CAD build for the part. Positions are in the model's coordinates, mm. A direction names the side the tool comes from. Round coordinates to 2 decimals unless told otherwise and drop trailing zeros. Order: outer loops, then holes, each group sorted by start corner. A loop starts at its lowest first (then second) coordinate and runs counter-clockwise, first axis right, second up. Notation, with made-up numbers: (59.25, 72) -> (100.25, 72) arc R27 ccw to (100.25, 106) -> close; hole circle Ø4 at (34.25, 85). An arc over 180 degrees is marked (long way). Return JSON: item names as keys, results as strings. Group by question number.
Q1. Probe line 1 along X through (y, z) = (62.5, -68.15); line 2 along Y through (x, z) = (35, -67.9); line 3 along Y through (x, z) = (41, -63.1). List the from-to ranges inside material, lowest first.
Q2. Mould opens along Y. For faces 6 (the flat face through (40, 1, -67)), 7 (the cylindrical face through (-35.962, 64.447, -66.014)), 8 (the cylindrical face through (-93, 62.6, -68.5)) say: +Y half, -Y half, draft (parallel to the pull), parting line (faces both ways), or undercut.
Q3. Cut at D-D (x = -27.5). Write the cut outline in (y, z), then the cut area to 3 significant figures.
Q4. Cut at C-C (x = 41). Write the cut outline in (y, z).
Q5. Cut at B-B (y = 68.5). Write the cut outline in (x, z), then the cut area to 3 significant figures.
Q6. Flat gauge pins, fed straight in: pin 1 (5.5 mm diameter, centred on x = 41, y = -68.5, fed in from +Z); pin 2 (5 mm diameter, centred on x = -90, y = 62.5, fed in from -Z); pin 3 (2 mm diameter, centred on x = 16, y = -37.5, fed in from +Z). Where does each tip first touch, or does it go through?
Q7. Which spindle directions (+Z, -Z, +X, -X, +Y, -Y) get a long thin tool onto all of the face, cutting with end or side? Do faces 1 (the flat face through (40, 1, -65)), 2 (the cylindrical face through (38.6, -70.3, -63.5)), 3 (the cylindrical face through (-71.722, 40.551, -66.028)), 4 (the flat face through (-63, 53, -62)), 5 (the cylindrical face through (-93, -62.4, -68.5)). Say none if no direction does.
Q8. Cut at A-A (y = 0). Write the cut outline in (x, z), then the cut area to 3 significant figures.
from build123d import *

# Parameters (mm, degrees)
CYLINDER058_R     = 3
CYLINDER058_DEPTH = 4
CYLINDER059_R     = 3
CYLINDER059_DEPTH = 4
CYLINDER060_R     = 3
CYLINDER060_DEPTH = 4
CYLINDER061_R     = 3
CYLINDER061_DEPTH = 4
CYLINDER062_R     = 3
CYLINDER062_DEPTH = 4
CYLINDER063_R     = 3
CYLINDER063_DEPTH = 4
CYLINDER064_R     = 3
CYLINDER064_DEPTH = 4
CYLINDER065_R     = 3
CYLINDER065_DEPTH = 4
CYLINDER056_R     = 60
CYLINDER056_DEPTH = 8
BOX015_W          = 155
BOX015_H          = 155
BOX015_DEPTH      = 3
CYLINDER057_R     = 65
CYLINDER057_DEPTH = 8
BOX016_W          = 155
BOX016_H          = 155
BOX016_DEPTH      = 3
FILLET008_R       = 2


with BuildPart() as cylinder086:
    # Cylinder058 → Cylinder058 (new body)
    with BuildSketch(Plane(origin=(35, 62.5, -30), x_dir=(1, 0, 0), z_dir=(0, 0, 1))):
        Circle(CYLINDER058_R)
    extrude(amount=CYLINDER058_DEPTH)


with BuildPart() as cylinder087:
    # Cylinder059 → Cylinder059 (new body)
    with BuildSketch(Plane(origin=(35, -62.5, -30), x_dir=(1, 0, 0), z_dir=(0, 0, 1))):
        Circle(CYLINDER059_R)
    extrude(amount=CYLINDER059_DEPTH)


with BuildPart() as cylinder088:
    # Cylinder060 → Cylinder060 (new body)
    with BuildSketch(Plane(origin=(-90, 62.5, -30), x_dir=(1, 0, 0), z_dir=(0, 0, 1))):
        Circle(CYLINDER060_R)
    extrude(amount=CYLINDER060_DEPTH)


with BuildPart() as lower_plate_screw_holes:
    # Cylinder061 → Cylinder061 (new body)
    with BuildSketch(Plane(origin=(-90, -62.5, -30), x_dir=(1, 0, 0), z_dir=(0, 0, 1))):
        Circle(CYLINDER061_R)
    extrude(amount=CYLINDER061_DEPTH)

    # Fusion025: union Cylinder086, Cylinder087, Cylinder088
    add(cylinder086.part)
    add(cylinder087.part)
    add(cylinder088.part)


with BuildPart() as cylinder090:
    # Cylinder062 → Cylinder062 (new body)
    with BuildSketch(Plane(origin=(41, -68.5, -26), x_dir=(1, 0, 0), z_dir=(0, 0, 1))):
        Circle(CYLINDER062_R)
    extrude(amount=CYLINDER062_DEPTH)


with BuildPart() as cylinder091:
    # Cylinder063 → Cylinder063 (new body)
    with BuildSketch(Plane(origin=(-96, 68.5, -26), x_dir=(1, 0, 0), z_dir=(0, 0, 1))):
        Circle(CYLINDER063_R)
    extrude(amount=CYLINDER063_DEPTH)


with BuildPart() as cylinder092:
    # Cylinder064 → Cylinder064 (new body)
    with BuildSketch(Plane(origin=(41, 68.5, -26), x_dir=(1, 0, 0), z_dir=(0, 0, 1))):
        Circle(CYLINDER064_R)
    extrude(amount=CYLINDER064_DEPTH)


with BuildPart() as obj1:
    # Cylinder065 → Cylinder065 (new body)
    with BuildSketch(Plane(origin=(-96, -68.5, -26), x_dir=(1, 0, 0), z_dir=(0, 0, 1))):
        Circle(CYLINDER065_R)
    extrude(amount=CYLINDER065_DEPTH)

    # Fusion026: union Cylinder090, Cylinder091, Cylinder092
    add(cylinder090.part)
    add(cylinder091.part)
    add(cylinder092.part)

    # Fusion027: union lower plate screw holes
    add(lower_plate_screw_holes.part)


with BuildPart() as cylinder084:
    # Cylinder056 → Cylinder056 (new body)
    with BuildSketch(Plane(origin=(77.5, 77.5, -30), x_dir=(1, 0, 0), z_dir=(0, 0, 1))):
        Circle(CYLINDER056_R)
    extrude(amount=CYLINDER056_DEPTH)


with BuildPart() as cube008:
    # Box015 → Box015 (new body)
    with BuildSketch(Plane.XY.offset(-25)):
        with Locations((77.5, 77.5)):
            Rectangle(BOX015_W, BOX015_H)
    extrude(amount=BOX015_DEPTH)


with BuildPart() as cylinder085:
    # Cylinder057 → Cylinder057 (new body)
    with BuildSketch(Plane(origin=(77.5, 77.5, -30), x_dir=(1, 0, 0), z_dir=(0, 0, 1))):
        Circle(CYLINDER057_R)
    extrude(amount=CYLINDER057_DEPTH)


with BuildPart() as obj2:
    # Box016 → Box016 (new body)
    with BuildSketch(Plane.XY.offset(-30)):
        with Locations((77.5, 77.5)):
            Rectangle(BOX016_W, BOX016_H)
    extrude(amount=BOX016_DEPTH)

    # Fusion024: union Cube008, Cylinder085
    add(cube008.part)
    add(cylinder085.part)

    # Cut022: cut Cylinder084
    add(cylinder084.part, mode=Mode.SUBTRACT)


with BuildPart() as obj2_1:
    # Cut022 placement: moved
    add(obj2.part.moved(Location((-105, -77.5, 0))))

    # Fillet008
    fillet008_edges = [obj2_1.edges().sort_by_distance(p)[0] for p in [
        (-87.5, 0, -22),
        (-87.5, 0, -30),
    ]]
    fillet(fillet008_edges, radius=FILLET008_R)

    # Cut023: cut obj1
    add(obj1.part, mode=Mode.SUBTRACT)


with BuildPart() as obj2_2:
    # Cut023 placement: moved
    add(obj2_1.part.moved(Location((0, 0, -40))))


solid = obj2_2.part
Solution:
{
 "1": {"line 1": "x = -105 to -93, -87 to 32, 38 to 50", "line 2": "y = -77.5 to -65.5, -59.5 to 59.5, 65.5 to 77.5", "line 3": "y = -77.5 to -71.5, -65.5 to 65.5, 71.5 to 77.5"},
 "2": {"face 6": "draft", "face 7": "parting line", "face 8": "undercut"},
 "3": {"outline": "(-77.5, -70) -> (-62, -70) arc R2 ccw to (-60, -68) -> (-60, -64) arc R2 ccw to (-62, -62) -> (-77.5, -62) -> (-77.5, -65) -> (-65, -65) -> (-65, -67) -> (-77.5, -67) -> close; (60, -68) arc R2 ccw to (62, -70) -> (77.5, -70) -> (77.5, -67) -> (65, -67) -> (65, -65) -> (77.5, -65) -> (77.5, -62) -> (62, -62) arc R2 ccw to (60, -64) -> close", "area": "227 mm²"},
 "4": {"outline": "(-77.5, -70) -> (77.5, -70) -> (77.5, -67) -> (-77.5, -67) -> close; (-77.5, -65) -> (-71.5, -65) -> (-71.5, -62) -> (-77.5, -62) -> close; (-65.5, -65) -> (65.5, -65) -> (65.5, -62) -> (-65.5, -62) -> close; (71.5, -65) -> (77.5, -65) -> (77.5, -62) -> (71.5, -62) -> close"},
 "5": {"outline": "(-105, -70) -> (50, -70) -> (50, -67) -> (-105, -67) -> close; (-105, -65) -> (-99, -65) -> (-99, -62) -> (-105, -62) -> close; (-93, -65) -> (38, -65) -> (38, -62) -> (-93, -62) -> close; (44, -65) -> (50, -65) -> (50, -62) -> (44, -62) -> close", "area": "894 mm²"},
 "6": {"pin 1": "stops at z = -67", "pin 2": "stops at z = -65", "pin 3": "passes through"},
 "7": {"face 1": "none", "face 2": "+Z", "face 3": "+Z, -Z", "face 4": "+Z, +X, -X, +Y, -Y", "face 5": "-Z"},
 "8": {"outline": "(-105, -70) -> (-89.5, -70) arc R2 ccw to (-87.5, -68) -> (-87.5, -64) arc R2 ccw to (-89.5, -62) -> (-105, -62) -> (-105, -65) -> (-92.5, -65) -> (-92.5, -67) -> (-105, -67) -> close; (32.5, -68) arc R2 ccw to (34.5, -70) -> (50, -70) -> (50, -67) -> (37.5, -67) -> (37.5, -65) -> (50, -65) -> (50, -62) -> (34.5, -62) arc R2 ccw to (32.5, -64) -> close", "area": "227 mm²"}
}
